Geometry: see drawing. Coordinates: mm, zero at the bounding-box minimum. A direction names the side the tool comes from. Give positions to 0.01 mm unless a question says otherwise; leave off trailing zeros. Loops run counter-clockwise (first coordinate to the right, second up) from the corner with the lowest first, then second, coordinate; pieces in that order, holes last. Notation, with made-up numbers: (11.5, 2.25) -> (65.5, 2.25) arc R24 ccw to (65.5, 29.25) -> close; hole circle Ø11 at (76, 26). An arc over 180 degrees is marked (long way). Use CSV: the item, a comma, the result in double quotes.
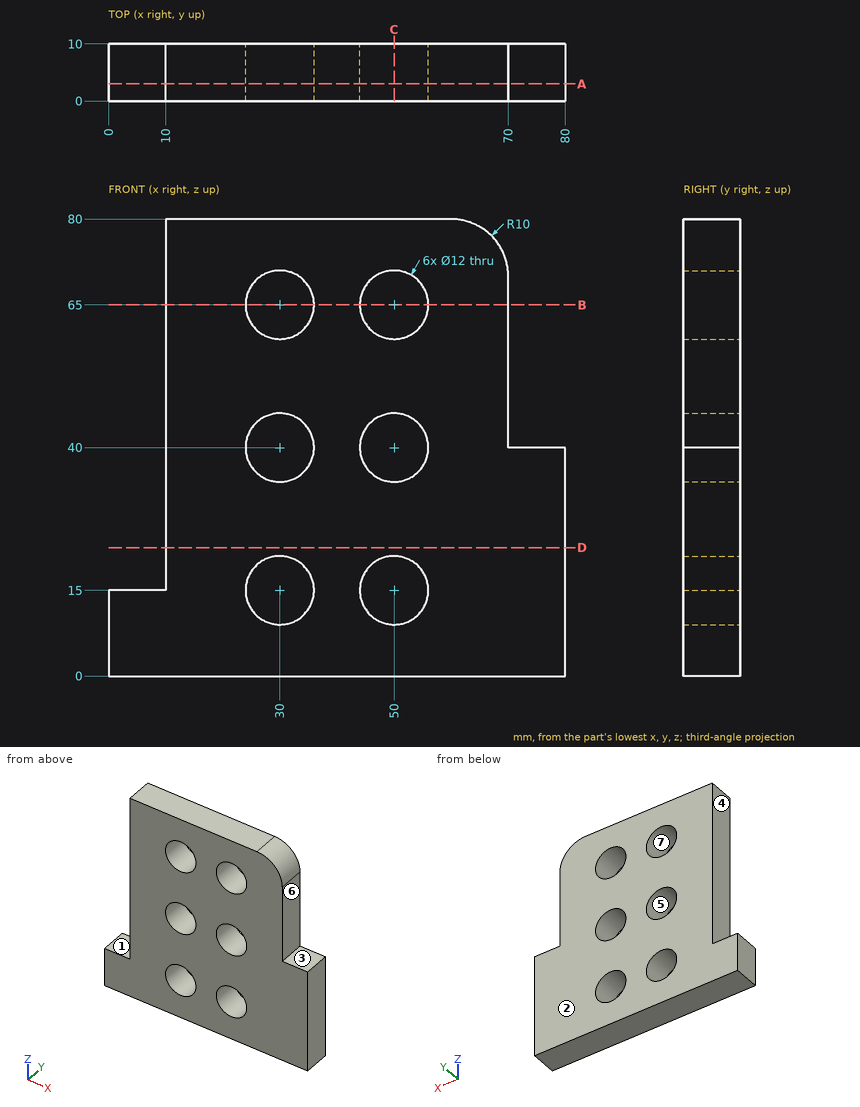
1) Mould query, pull axis X, two halves, no side actions, for the marked faces 4, 5, 6 and 7. Classes: pulls with the +X half, pulls with the -X half, needs draft (parallel to the pull), parting line crosses it, or undercut.
From the geometry:
face 4,"pulls with the -X half"
face 5,"undercut"
face 6,"pulls with the +X half"
face 7,"undercut"
2) Section query C-C (x = 50). Return loops of the section in (y, z), then the cut area to 3 significant figures.
From the geometry:
outline,"(0, 0) -> (10, 0) -> (10, 9) -> (0, 9) -> close; (0, 21) -> (10, 21) -> (10, 34) -> (0, 34) -> close; (0, 46) -> (10, 46) -> (10, 59) -> (0, 59) -> close; (0, 71) -> (10, 71) -> (10, 80) -> (0, 80) -> close"
area,"440 mm^2"
3) Section query D-D (z = 22.5). Return loops of the section in (x, y), then the cut area to 3 significant figures.
From the geometry:
outline,"(10, 0) -> (80, 0) -> (80, 10) -> (10, 10) -> close"
area,"700 mm^2"
4) Ray query, line 1 (Z direction, x = 30, y = 4.75); line 2 (Z direction, x = 28, y = 1.5); line 3 (X direction, y = 6.75, z = 19.5). Return the intervals inside material, ascending.
From the geometry:
line 1,"z = 0 to 9, 21 to 34, 46 to 59, 71 to 80"
line 2,"z = 0 to 9.34, 20.66 to 34.34, 45.66 to 59.34, 70.66 to 80"
line 3,"x = 10 to 26.03, 33.97 to 46.03, 53.97 to 80"
5) Section query B-B (z = 65). Return loops of the section in (x, y), then the cut area to 3 significant figures.
From the geometry:
outline,"(10, 0) -> (24, 0) -> (24, 10) -> (10, 10) -> close; (36, 0) -> (44, 0) -> (44, 10) -> (36, 10) -> close; (56, 0) -> (70, 0) -> (70, 10) -> (56, 10) -> close"
area,"360 mm^2"
6) Section query A-A (y = 3). Return loops of the section in (x, z).
From the geometry:
outline,"(0, 0) -> (80, 0) -> (80, 40) -> (70, 40) -> (70, 70) arc R10 ccw to (60, 80) -> (10, 80) -> (10, 15) -> (0, 15) -> close; hole circle Ø12 at (30, 15); hole circle Ø12 at (30, 40); hole circle Ø12 at (30, 65); hole circle Ø12 at (50, 15); hole circle Ø12 at (50, 40); hole circle Ø12 at (50, 65)"
7) Contact query for flat-ended pins moving along their axis: pin 1 (5 mm diameter, centred on y = 6, z = 49.5, fed in from +X); pin 2 (9.5 mm diameter, centred on x = 50, z = 40, fed in from +Y); pin 3 (4 mm diameter, centred on y = 1, z = 62, fed in from -X); pin 4 (3 mm diameter, centred on x = 73, y = 3, fed in from +Z). Output: stop coordinate, or through.
From the geometry:
pin 1,"stops at x = 70"
pin 2,"passes through"
pin 3,"stops at x = 10"
pin 4,"stops at z = 40"
8) Reachability of the marked faces 1, 2 and 3 from +Z, -Z, +X, -X, +Y, -Y: full face, straight path, thin tool, end or side. Return the list, or none.
From the geometry:
face 1,"+Z, -X, +Y, -Y"
face 2,"+Z, -Z, +X, -X, +Y"
face 3,"+Z, +X, +Y, -Y"
